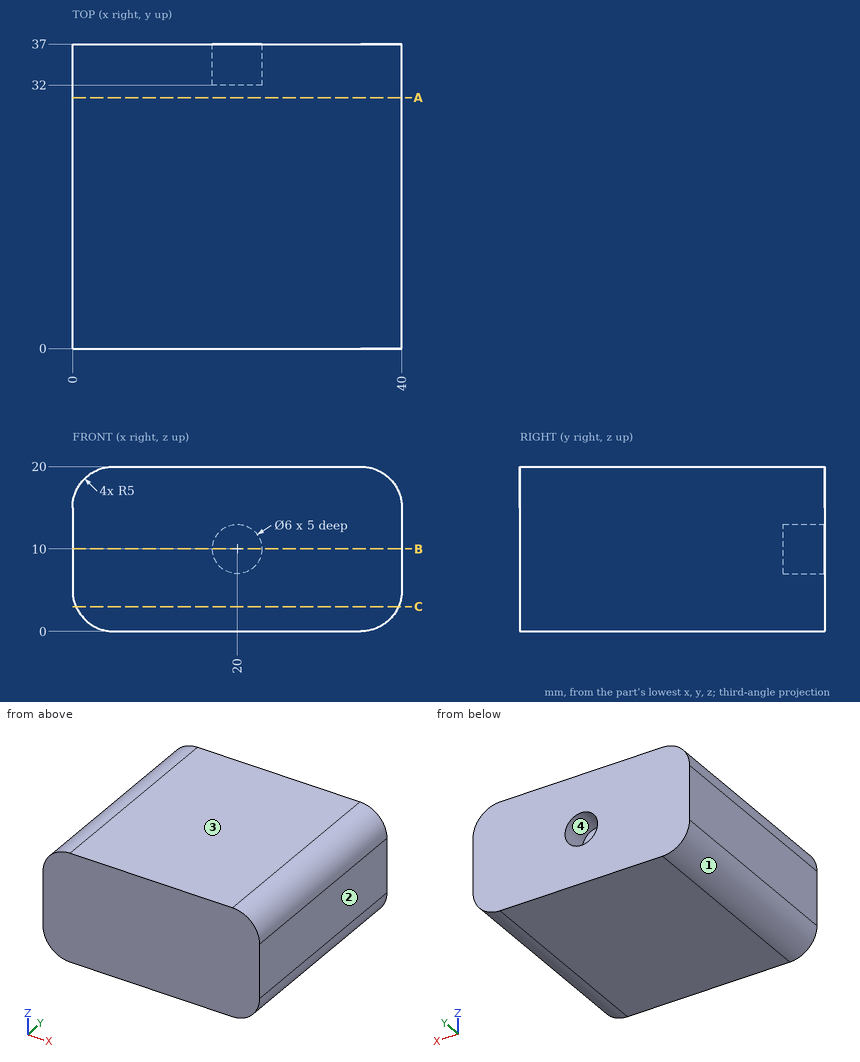
Here's the drawing with two shaded views (mm, measured from the low corner). I have some questions. Coordinates: 2 decimals unless noted, no trailing zeros. Loops run counter-clockwise (first coordinate to the right, second up) from the corner with the lowest first, then second, coordinate; pieces in that order, holes last. Notation, with made-up numbers: M 15,48.25 L 31,48.25 A19 ccw 31,79.25 Z; hole C 32,-23 d9. An arc over 180 degrees is marked long. Answer as CSV lines item,"result". Start each with the question number.
1. Suppose I cut it at C-C, the plane z = 3. List the corners of the cut face in (x, y) for me, plus the area to 3 significant figures.
2. Thinking about a two-plate mould opening in Z: for the marked faces 1, 2, 3 and 4, which applies, +Z half, -Z half, draft (parallel to the pull), parting line (faces both ways), or undercut?
3. For pin 1 Ø6.5 at (x, z) = (18.5, 9.5) entering from +Y, with a flat end and sliding along its axis, tell me the tip position at first contact or that it passes through.
4. Suppose I cut it at B-B, the plane z = 10. List the corners of the cut face in (x, y) for me.
5. Suppose I cut it at A-A, the plane y = 30.5. List the corners of the cut face in (x, z) for me, plus the area to 3 significant figures.
6. If I drill on probe 1 along X at (y, z) = (33.5, 10); probe 2 along Z at (x, y) = (20, 33.2); probe 3 along X at (y, z) = (32.5, 8), over which ranges is the centre line in solid material (lowest first)? Write a range as [from, to].
Output:
1,outline,"M 0.42,0 L 39.58,0 L 39.58,37 L 0.42,37 Z"
1,area,"1,450 mm^2"
2,face 1,"-Z half"
2,face 2,"draft"
2,face 3,"+Z half"
2,face 4,"undercut"
3,pin 1,"stops at y = 37"
4,outline,"M 0,0 L 40,0 L 40,37 L 23,37 L 23,32 L 17,32 L 17,37 L 0,37 Z"
5,outline,"M 0,5 A5 ccw 5,0 L 35,0 A5 ccw 40,5 L 40,15 A5 ccw 35,20 L 5,20 A5 ccw 0,15 Z"
5,area,"779 mm^2"
6,probe 1,"x = [0, 17], [23, 40]"
6,probe 2,"z = [0, 7], [13, 20]"
6,probe 3,"x = [0, 17.76], [22.24, 40]"
